from build123d import *

# Parameters (mm, degrees)
F1_DEPTH = 300
F2_R     = 70
F4_DEPTH = 1454


with BuildPart() as f1:
    # F0 (on Front) → F1 (new body)
    with BuildSketch(Plane.XZ):
        with BuildLine():
            Line((-280, -300), (280.009727, -300))
            ThreePointArc((280.009727, -300), (330.254635, -278.73858), (349.977312, -227.869977))
            Line((349.977312, -227.869977), (350, 200))
            ThreePointArc((350, 200), (320.710678, 270.710678), (250, 300))
            Line((250, 300), (100, 300))
            Line((100, 300), (100, 1200))
            Line((100, 1200), (-100, 1200))
            Line((-100, 1200), (-100, 300))
            Line((-100, 300), (-280, 300))
            ThreePointArc((-280, 300), (-329.497475, 279.497475), (-350, 230))
            Line((-350, 230), (-350, -230))
            ThreePointArc((-350, -230), (-329.497475, -279.497475), (-280, -300))
        make_face()
        Polygon((-250, 100), (-250, 200), (250, 200), (250, 100), (150, 100), (150, -100), (250, -100), (249.994698, -200), (-250, -200), (-250, -100), (-150, -100), (-150, 100), align=None, mode=Mode.SUBTRACT)
    extrude(amount=F1_DEPTH)

    # F2
    f2_edges = [f1.edges().sort_by_distance(p)[0] for p in [
        (0, 0, 1200),
        (0, -300, 1200),
    ]]
    fillet(f2_edges, radius=F2_R)


with BuildPart() as f4:
    # F3 (on face) → F4 (new body)
    with BuildSketch(Plane.YZ.offset(100)):
        with BuildLine():
            Line((-100, 400.005119), (-100.071387, 1097.329122))
            ThreePointArc((-100.071387, 1097.329122), (-148.884053, 1149.987545), (-199.998063, 1099.559935))
            Line((-199.998063, 1099.559935), (-200, 400.000138))
            ThreePointArc((-200, 400.000138), (-149.99751, 350), (-100, 400.005119))
        make_face()
    extrude(amount=-F4_DEPTH)


with BuildPart() as f1_1:
    add(f1.part)

    # F5: cut F4
    add(f4.part, mode=Mode.SUBTRACT)


solid = f1_1.part
Here's how the part is built. I have some questions about the finished solid (model axes, mm). A direction names the side the tool comes from. Give positions to 0.01 mm unless a question says otherwise; leave off trailing zeros. Order: outer loops, then holes, each group sorted by start corner. A loop starts at its lowest first (then second) coordinate and runs counter-clockwise, first axis right, second up. Notation, with made-up numbers: M 52.25,-9 L 82.25,-9 A14 cw 82.25,-2 Z; hole C 53.5,-15.75 d2. An arc over 180 degrees is marked long. Answer as a JSON object with one key per item and string values. Group by question number.
1) Please list where these lines run through material, in increasing order: L1, parallel to Z at x = 167.5, y = -95.5; L2, parallel to X at y = -244, z = 191.5; L3, parallel to Y at x = 38.5, z = 736. Write a range as [from, to].
2) Suppose I cut it at A-A, the plane y = -150. Write out the boundary of the cut face in (x, z).
3) Suppose I cut it at D-D, the plane z = 1009.5. Write out the boundary of the cut face in (x, y).
4) I'm going to push flat-ended pins straight in: pin 1 Ø10 at (x, y) = (68.5, -264.5) entering from +Z; pin 2 Ø1 at (x, z) = (-165.5, -30.5) entering from +Y. Where does each tip first touch, or does it pass through?
5) Suppose I cut it at C-C, the plane x = 47. Write out the boundary of the cut face in (y, z), plus the area to 3 significant figures.
6) On a 3-axis mill with a long thin cutter (end or side, diameter ignored), from which of +Z, -Z, +X, -X, +Y, -Y can I reach the whole of each face in a straight line? I mean faces 1 (the cylindrical face through (1.4, -147.76, 1149.95)), 2 (the flat face through (3, -148, -200)), 3 (the flat face through (-189, -148, 300)). Say none if no direction works.
7) Suppose I cut it at B-B, the plane x = -126. Write out the boundary of the cut face in (y, z).
8) We'd pull the mould along X, two halves only. Please class faces 4 (the cylindrical face through (-1.4, -278.95, 1180.04)), 5 (the flat face through (-350, -148, 3)), 6 (the flat face through (-3, -148, 200)), 7 (the flat face through (250, -148, 151)): pulls with the +X half, pulls with the -X half, needs draft (parallel to the pull), parting line crosses it, or undercut.
Results found:
{
 "1": {"L1": "[-300, -200], [-100, 100], [200, 300]", "L2": "[-350, -250], [250, 350]", "L3": "[-300, -200], [-100.03, 0]"},
 "2": {"outline": "M -350,-230 A70 ccw -280,-300 L 280.01,-300 A70 ccw 349.98,-227.87 L 350,200 A100 ccw 250,300 L 100,300 L 100,350 L -100,350 L -100,300 L -280,300 A70 ccw -350,230 Z; M -100,1150 L 100,1150 L 100,1200 L -100,1200 Z; hole M -250,-200 L 249.99,-200 L 250,-100 L 150,-100 L 150,100 L 250,100 L 250,200 L -250,200 L -250,100 L -150,100 L -150,-100 L -250,-100 Z"},
 "3": {"outline": "M -100,-300 L 100,-300 L 100,-200 L -100,-200 Z; M -100,-100.06 L 100,-100.06 L 100,0 L -100,0 Z"},
 "4": {"pin 1": "z = 1193.48", "pin 2": "y = 0"},
 "5": {"outline": "M -300,-300 L 0,-300 L 0,-200 L -300,-200 Z; M -300,200 L 0,200 L 0,1130 A70 ccw -70,1200 L -230,1200 A70 ccw -300,1130 Z; hole M -200,400 A50 ccw -100,400.01 L -100.07,1097.33 A50 ccw long -200,1099.56 Z", "area": "250,000 mm²"},
 "6": {"face 1": "+X, -X", "face 2": "+Y, -Y", "face 3": "+Z, -X, +Y, -Y"},
 "7": {"outline": "M -300,-300 L 0,-300 L 0,-200 L -300,-200 Z; M -300,200 L 0,200 L 0,300 L -300,300 Z"},
 "8": {"face 4": "needs draft", "face 5": "pulls with the -X half", "face 6": "undercut", "face 7": "undercut"}
}
